Autodesk Inventor part; units mm, degrees
ref_plane "YZ Plane" through (0, 0, 0) normal (1, 0, 0) x (0, 1, 0)
ref_plane "XZ Plane" through (0, 0, 0) normal (0, 1, 0) x (-1, 0, 0)
ref_plane "XY Plane" through (0, 0, 0) normal (0, 0, 1) x (1, 0, 0)
sketch "Sketch1" plane through (0, 0, 0) normal (0, 1, 0) x (-1, 0, 0)
  line L0 (0, 0) -> (58, 0) construction
  line L1 (58, 0) -> (58, -48) construction
  line L2 (58, -48) -> (0, -48) construction
  line L3 (0, -48) -> (0, 0) construction
  circle A0 centre (50.5, -7.5) radius 2.35
  circle A1 centre (50.5, -40.5) radius 2.35
  circle A2 centre (7.5, -7.5) radius 2.35
  circle A3 centre (7.5, -40.5) radius 2.35
  circle A4 centre (50.5, -7.5) radius 5
  circle A5 centre (50.5, -40.5) radius 5
  circle A6 centre (7.5, -7.5) radius 5
  circle A7 centre (7.5, -40.5) radius 5
  dimension "d0" = 58
  dimension "d1" = 48
  dimension "d2" = 4.7
  dimension "d3" = 4.7
  dimension "d4" = 4.7
  dimension "d5" = 4.7
  dimension "d6" = 33
  dimension "d7" = 43
  dimension "d8" = 7.5
  dimension "d9" = 7.5
  dimension "d10" = 7.5
  dimension "d11" = 7.5
  dimension "d12" = 7.5
  dimension "d13" = 7.5
  dimension "d14" = 10
  dimension "d15" = 10
  dimension "d16" = 10
  dimension "d17" = 10
extrude "Extrusion1" add sketch "Sketch1" along normal blind 12
sketch "Sketch2" plane through (-50.5, 12, -7.5) normal (0, 1, 0) x (1, 0, 0)
  line L0 (-31, -18.5) -> (74, -18.5)
  line L1 (74, -18.5) -> (74, 51.5)
  line L2 (74, 51.5) -> (-31, 51.5)
  line L3 (-31, 51.5) -> (-31, -18.5)
  circle A0 centre (0, 0) radius 2.35
  circle A1 centre (0, 33) radius 2.35
  circle A2 centre (43, 33) radius 2.35
  circle A3 centre (43, 0) radius 2.35
  circle A4 centre (43, 0) radius 2.35
  point P0 (50.5, -7.5)
  dimension "d20" = 105
  dimension "d21" = 70
  dimension "d22" = 18.5
  dimension "d23" = 31
extrude "Extrusion3" add sketch "Sketch2" along normal blind 4
sketch "Sketch3" plane through (-50.5, 16, -7.5) normal (0, 1, 0) x (1, 0, 0)
  line L0 (-31, 51.5) -> (-31, -18.5)
  line L1 (-31, -18.5) -> (-31, 1.5)
  line L2 (-31, 1.5) -> (-28, 1.5)
  line L3 (-28, 1.5) -> (-28, -15.5)
  line L4 (-28, -15.5) -> (-11, -15.5)
  line L5 (-11, -15.5) -> (-11, -18.5)
  line L6 (-11, -18.5) -> (-31, -18.5)
  line L7 (-28, 48.5) -> (-11, 48.5)
  line L8 (-11, 48.5) -> (-11, 51.5)
  line L9 (74, -18.5) -> (74, 51.5)
  line L10 (74, 51.5) -> (54, 51.5)
  line L11 (54, 51.5) -> (54, 48.5)
  line L12 (71, 31.5) -> (74, 31.5)
  line L13 (74, 31.5) -> (74, 51.5)
  line L14 (74, -18.5) -> (74, 1.5)
  line L15 (74, 1.5) -> (71, 1.5)
  line L16 (71, 1.5) -> (71, -15.5)
  line L17 (71, -15.5) -> (54, -15.5)
  line L18 (54, -15.5) -> (54, -18.5)
  line L19 (54, -18.5) -> (74, -18.5)
  line L20 (74, 51.5) -> (-31, 51.5)
  line L21 (54, 48.5) -> (71, 48.5)
  line L22 (71, 48.5) -> (71, 31.5)
  line L23 (-11, 51.5) -> (-31, 51.5)
  line L24 (-31, 51.5) -> (-31, 41.5)
  line L25 (-31, 41.5) -> (-28, 41.5)
  line L26 (-28, 41.5) -> (-28, 48.5)
  point P0 (50.5, -7.5)
  dimension "d28" = 20
  dimension "d37" = 3
  dimension "d48" = 20
  dimension "d49" = 3
  dimension "d50" = 3
  dimension "d51" = 3
  dimension "d52" = 3
  dimension "d53" = 20
  dimension "d54" = 20
  dimension "d55" = 20
  dimension "d56" = 20
  dimension "d57" = 3
  dimension "d58" = 3
  dimension "d69" = 10
  dimension "d70" = 7
extrude "Extrusion4" add sketch "Sketch3" along normal blind 28
fillet "Fillet1" radius 10 7 edges at (-61.5, 16, 9.5) (-80, 16, -9) (-61.5, 16, -57.5) (3.5, 16, -57.5) (22, 16, -39) (22, 16, -9) (3.5, 16, 9.5)
sketch "Sketch4" plane through (-81.5, 12, 11) normal (0, 0, 1) x (1, 0, 0)
  line L0 (0, 0) -> (0, 32)
  line L1 (0, 0) -> (100, 0)
  line L2 (100, 0) -> (100, -15)
  line L3 (100, -15) -> (0, -15)
  line L4 (0, -15) -> (0, 0)
  point P0 (81.5, -12)
  dimension "d59" = 100
  dimension "d60" = 15
extrude "remove legs" cut sketch "Sketch4" against normal through all
sketch "Sketch5" plane through (-50.5, 12, -7.5) normal (0, -1, 0) x (1, 0, 0)
  circle A0 centre (0, 0) radius 2.35
  circle A1 centre (0, 0) radius 4.1
  circle A2 centre (43, 0) radius 2.35
  circle A3 centre (43, 0) radius 4.1
  circle A4 centre (43, -33) radius 2.35
  circle A5 centre (43, -33) radius 4.1
  circle A6 centre (0, -33) radius 2.35
  circle A7 centre (0, -33) radius 4.1
  circle A8 centre (0, 0) radius 2.35
  circle A9 centre (43, 0) radius 2.35
  circle A10 centre (43, -33) radius 2.35
  circle A11 centre (0, -33) radius 2.35
  point P0 (50.5, 7.5)
  dimension "d63" = 8.2
  dimension "d64" = 8.2
  dimension "d65" = 8.2
  dimension "d66" = 8.2
extrude "Extrusion6" cut sketch "Sketch5" against normal blind 4
fillet "Fillet2" radius 4 1 edges at (-80, 16, -49)
properties part number "TestingPlatform_base01"
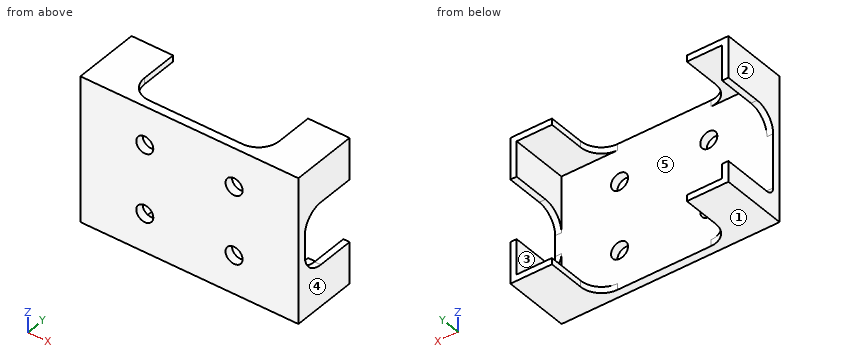
The model under review builds one solid part; all positions refer to its coordinate system, in mm. Face numbers are marked on the shaded views. A direction names the side the tool comes from. Give positions to 0.01 mm unless a question says otherwise; leave off trailing zeros. Write each loop counter-clockwise with the first axis right and the second up, starting at its lowest first coordinate (ties: lowest second). Pieces come first, ordered by that corner, then holes. Notation, with made-up numbers: M 17.5,-38 L 42.5,-38 A36 ccw 42.5,-1 Z; hole C 57.25,83 d11. An arc over 180 degrees is marked long. One line per question, with ' | ' between items. Start each with the question number.
Item 1: We need section B-B on y = 39. Write out the cut boundary in (x, z), plus the area to 3 significant figures.
Item 2: Draft analysis for pull direction X (two halves, no side actions). For the marked faces 1, 2 and 3, state which applies: released by +X, released by -X, zero draft, split by the parting line, or undercut.
Item 3: We need section A-A on z = -40.5. Write out the cut boundary in (x, y), plus the area to 3 significant figures.
Item 4: We need section C-C on x = 7. Write out the cut boundary in (y, z), plus the area to 3 significant figures.
Item 5: Wall thickness on line 1 (Z direction, x = 18, y = 19.5); line 2 (X direction, y = 15, z = -7); line 3 (Z direction, x = -7.5, y = 14.15): over which ranges is each line inside the solid? List them lowest first. Write a range as from..to.
Item 6: For the marked faces 4 and 5, list the 3-axis set-ups (+Z, -Z, +X, -X, +Y, -Y) from which the entire face can be reached by the end or side of a thin tool; tool diameter is ignored.
Item 7: For pin 1 (13.5 mm diameter, centred on y = 29, z = -36.5, fed in from -X); pin 2 (3 mm diameter, centred on x = 11, z = -3, fed in from +Y), all flat-tipped, find the tip position at first contact; note any pin that passes through.
Item 8: We need section D-D on z = -7.5. Write out the cut boundary in (x, y).
Results found:
1) outline: M -81.5,-59 L -61.5,-59 L -61.5,-56 L -78.5,-56 L -78.5,-49 L -81.5,-49 Z; M -81.5,-9 L -78.5,-9 L -78.5,8 L -61.5,8 L -61.5,11 L -81.5,11 Z; M 3.5,-59 L 23.5,-59 L 23.5,-39 L 20.5,-39 L 20.5,-56 L 3.5,-56 Z; M 3.5,8 L 20.5,8 L 20.5,-9 L 23.5,-9 L 23.5,11 L 3.5,11 Z | area: 414 mm2
2) face 1: zero draft | face 2: released by -X | face 3: undercut
3) outline: M -81.5,12 L -54.6,12 L -54.6,16 L -81.5,16 Z; M -46.4,12 L -11.6,12 L -11.6,16 L -46.4,16 Z; M -3.4,12 L 23.5,12 L 23.5,44 L 20.5,44 L 20.5,16 L -3.4,16 Z | area: 438 mm2
4) outline: M 12,-59 L 44,-59 L 44,-56 L 16,-56 L 16,8 L 44,8 L 44,11 L 12,11 Z | area: 448 mm2
5) line 1: z = -59..-56, 8..11 | line 2: x = -81.5..-54.57, -46.43..-11.57, -3.43..23.5 | line 3: z = -59..-44.6, -36.4..-11.6, -3.4..11
6) face 4: +Z, -Z, +X, +Y, -Y | face 5: +Y
7) pin 1: stops at x = 20.5 | pin 2: stops at y = 16
8) outline: M -81.5,12 L -54.6,12 L -54.6,16 L -78.5,16 L -78.5,44 L -81.5,44 Z; M -46.4,12 L -11.6,12 L -11.6,16 L -46.4,16 Z; M -3.4,12 L 23.5,12 L 23.5,44 L 20.5,44 L 20.5,16 L -3.4,16 Z
